For this review, take the finished solid that the model builds, in its own axes (mm). A direction names the side the tool comes from. Coordinates: 2 decimals unless noted, no trailing zeros. Loops run counter-clockwise (first coordinate to the right, second up) from the corner with the lowest first, then second, coordinate; pieces in that order, holes last. Notation, with made-up numbers: M 27.25,8 L 40.25,8 A32 cw 40.25,41 Z; hole C -3.5,64.25 d5. An arc over 180 degrees is marked long. Answer as a JSON object with one key per item and string values. Group by question number.
Item 1: Insertion check: pin 1 (2 mm diameter, centred on y = 7.5, z = 4.5, fed in from +X); pin 2 (5 mm diameter, centred on x = 94.5, z = 35.5, fed in from -Y); pin 3 (5 mm diameter, centred on y = 8.5, z = 9.5, fed in from -X). Each pin has a flat end and moves straight along its axis. Give the tip position at first contact, or say it passes through.
Item 2: Mouldability with a two-part tool opening along X and no side actions: class faces 6 (the face through (75.591, -17.605, 41.399)), 7 (the face through (100.17, -0.4, 19.72)), 8 (the face through (98.17, -0.36, 20.71)) as +X half, -X half, draft (parallel to the pull), parting line (faces both ways), or undercut.
Item 3: Add section C-C (z = 8). State the section outline as (x, y) points (3 decimals), then the cut area to 3 significant figures.
Item 4: Add section B-B (z = 25). State the section outline as (x, y) points (3 decimals).
Item 5: Tool access review of faces 1 (the face through (75, 16.175, 21)), 2 (the face through (82, -23, 20)), 3 (the face through (50.83, 0.4, 19.72)), 4 (the face through (75, -23, 40)), 5 (the face through (76.886, -23.105, 31.425)): name each direction out of +Z, -Z, +X, -X, +Y, -Y from which nothing blocks a thin tool from reaching the whole face with its end or side.
Item 6: Add section A-A (x = 75.5). State the section outline as (y, z) points (3 decimals).
Item 7: Wall thickness on L1, parallel to Z at x = 75.5, y = -22.25; L2, parallel to Y at x = 74.5, z = 21.5 (3 decimals); L3, parallel to Z at x = 75, y = -23: over which ranges is each line inside the solid? List them lowest first. Write a range as from..to.
from build123d import *

# Parameters (mm, degrees)
PAD005_DEPTH    = 40
THICKNESS001_T  = 2
POCKET001_DEPTH = 5
SKETCH006_W     = 13
SKETCH006_H     = 40
SKETCH006_R     = 1.5
PAD006_DEPTH    = 10


with BuildPart() as part:
    # Sketch005 → Pad005 (new body)
    with BuildSketch(Plane.XY):
        with BuildLine():
            ThreePointArc((0, 16.175), (-16.175, 0), (0, -16.175))
            Line((0, -16.175), (13, -16.175))
            ThreePointArc((13, -16.175), (29.175, 0), (13, 16.175))
            Line((0, 16.175), (13, 16.175))
        make_face()
    extrude(amount=PAD005_DEPTH)

    # Thickness001
    thickness001_openings = [part.faces().sort_by_distance(p)[0] for p in [
        (6.5, 0, 0),
    ]]
    offset(amount=THICKNESS001_T, openings=thickness001_openings)

    # Thickness001 Face5 → Pocket001 (cut)
    with BuildSketch(Plane(origin=(6.5, 0, 40), x_dir=(0, -1, 0), z_dir=(0, 0, -1))):
        with BuildLine():
            ThreePointArc((16.175, 6.5), (0, 22.675), (-16.175, 6.5))
            Line((-16.175, 6.5), (-16.175, -6.5))
            ThreePointArc((-16.175, -6.5), (0, -22.675), (16.175, -6.5))
            Line((16.175, -6.5), (16.175, 6.5))
        make_face()
    extrude(amount=-POCKET001_DEPTH, mode=Mode.SUBTRACT)

    # Sketch006 (on Face12 of Pocket001) → Pad006 (join)
    with BuildSketch(Plane.XZ.offset(18.175)):
        with Locations((6.5, 20)):
            Rectangle(SKETCH006_W, SKETCH006_H)
        with Locations((6.5, 32)):
            Circle(SKETCH006_R, mode=Mode.SUBTRACT)
        with Locations((6.5, 20)):
            Circle(SKETCH006_R, mode=Mode.SUBTRACT)
        with Locations((6.5, 8)):
            Circle(SKETCH006_R, mode=Mode.SUBTRACT)
    extrude(amount=PAD006_DEPTH)


with BuildPart() as part_1:
    # Body002 placement: moved
    add(part.part.moved(Location((69, 0, 0))))


solid = part_1.part
From the geometry:
{
 "1": {"pin 1": "stops at x = 98.97", "pin 2": "stops at y = -15.18", "pin 3": "stops at x = 51.84"},
 "2": {"face 6": "draft", "face 7": "+X half", "face 8": "undercut"},
 "3": {"outline": "M 69,-28.175 L 74,-28.175 L 74,-18.175 L 77,-18.175 L 77,-28.175 L 82,-28.175 L 82,-18.175 A18.175 ccw 82,18.175 L 69,18.175 A18.175 ccw 69,-18.175 Z; hole M 69,-16.175 L 82,-16.175 A16.175 ccw 82,16.175 L 69,16.175 A16.175 ccw Z", "area": "368 mm²"},
 "4": {"outline": "M 69,-28.175 L 82,-28.175 L 82,-18.175 A18.175 ccw 82,18.175 L 69,18.175 A18.175 ccw 69,-18.175 Z; hole M 69,-16.175 L 82,-16.175 A16.175 ccw 82,16.175 L 69,16.175 A16.175 ccw Z"},
 "5": {"face 1": "+Z, -Z", "face 2": "+Z, -Z, +X, -Y", "face 3": "+Z, -Z, -X", "face 4": "+Z, +X, -X, -Y", "face 5": "-Y"},
 "6": {"outline": "M -28.175,0 L -16.175,0 L -16.175,42 A2 ccw -18.175,40 L -28.175,40 L -28.175,33.5 L -18.175,33.5 L -18.175,30.5 L -28.175,30.5 L -28.175,21.5 L -18.175,21.5 L -18.175,18.5 L -28.175,18.5 L -28.175,9.5 L -18.175,9.5 L -18.175,6.5 L -28.175,6.5 Z; M 16.175,0 L 18.175,0 L 18.175,40 A2 ccw 16.175,42 Z"},
 "7": {"L1": "z = 0..6.5, 9.5..18.5, 21.5..30.5, 33.5..40", "L2": "y = -28.175..-16.175, 16.175..18.175", "L3": "z = 0..6.59, 9.41..18.59, 21.41..30.59, 33.41..40"}
}
